Geometry: final body of the model. Coordinates: model frame, mm. A direction names the side the tool comes from. Round coordinates to 2 decimals unless told otherwise and drop trailing zeros. Loops run counter-clockwise (first coordinate to the right, second up) from the corner with the lowest first, then second, coordinate; pieces in that order, holes last. Notation, with made-up numbers: (26, 6) - (63, 6) arc R16 cw to (63, 16) - close; hole circle Ø5 at (-9.5, 58). An arc over 180 degrees is marked (long way). Write item = value, one per line. Start each with the question number.
Item 1: Section A-A (x = 6). Return loops of the section in (y, z), plus the area to 3 significant figures.
Item 2: Draft query along Z for faces 1 (the flat face through (2, -5, 2.2)), 2 (the flat face through (-3, -6, 1.8)), 3 (the cylindrical face through (0.06, 7.15, 0.89)). Return one class per face: pulls with the +Z half, pulls with the -Z half, needs draft (parallel to the pull), parting line crosses it, or undercut.
Item 3: Section D-D (y = 0). Return loops of the section in (x, z).
Item 4: Access query for faces 4 (the flat face through (6.656, -4.209, 0.887)), 5 (the cylindrical face through (2.4, -4.5, 3.8)), 6 (the cylindrical face through (-5, -3.83, 6.04)). Directions: +Z, -Z, +X, -X, +Y, -Y. A direction counts if a zero-diameter tool reaches every point of the face in a straight line with its end or side. Return the directions, or none.
Item 5: Line query: line 1 (Z direction, x = -5.5, y = 2.25); line 2 (Z direction, x = -6.25, y = -4); line 3 (Y direction, x = -8.5, z = 1.25). Output: solid intervals per line, ascending. Write a range as from..to.
Item 6: Section B-B (y = 5.75). Return loops of the section in (x, z) (3 decimals), plus the area to 3 significant figures.
Item 7: Section C-C (x = 0). Return loops of the section in (y, z).
from build123d import *

# Parameters (mm, degrees)
PAD_DEPTH    = 1.8
SKETCH001_R  = 6.3
PAD001_DEPTH = 0.4
SKETCH002_R  = 5.1
PAD002_DEPTH = 3.3
SKETCH003_R  = 6.3
PAD003_DEPTH = 1.1


with BuildPart() as part:
    # Sketch → Pad (new body)
    with BuildSketch(Plane.XY):
        with BuildLine():
            ThreePointArc((3.885224, 6.002294), (0, 7.15), (-3.885224, 6.002294))
            Line((-9.35, 2.465), (-3.885224, 6.002294))
            Line((-9.35, -2.465), (-9.35, 2.465))
            Line((-3.885224, -6.002294), (-9.35, -2.465))
            ThreePointArc((-3.885224, -6.002294), (0, -7.15), (3.885224, -6.002294))
            Line((9.35, -2.465), (3.885224, -6.002294))
            Line((9.35, 2.465), (9.35, -2.465))
            Line((3.885224, 6.002294), (9.35, 2.465))
        make_face()
    extrude(amount=PAD_DEPTH)

    # Sketch001 (on Face5 of Pad003) → Pad001 (join)
    with BuildSketch(Plane.XY.offset(1.8)):
        Circle(SKETCH001_R)
    extrude(amount=PAD001_DEPTH)

    # Sketch002 (on Face12 of Pad001) → Pad002 (join)
    with BuildSketch(Plane.XY.offset(2.2)):
        Circle(SKETCH002_R)
    extrude(amount=PAD002_DEPTH)

    # Sketch003 (on Face14 of Pad002) → Pad003 (join)
    with BuildSketch(Plane.XY.offset(5.5)):
        Circle(SKETCH003_R)
    extrude(amount=PAD003_DEPTH)


solid = part.part
Taken from the geometry:
q1.outline = (-4.63, 0) - (4.63, 0) - (4.63, 1.8) - (1.92, 1.8) - (1.92, 2.2) - (-1.92, 2.2) - (-1.92, 1.8) - (-4.63, 1.8) - close; (-1.92, 5.5) - (1.92, 5.5) - (1.92, 6.6) - (-1.92, 6.6) - close
q1.area = 22.4 mm^2
q2.face_1 = undercut
q2.face_2 = pulls with the +Z half
q2.face_3 = needs draft
q3.outline = (-9.35, 0) - (9.35, 0) - (9.35, 1.8) - (6.3, 1.8) - (6.3, 2.2) - (5.1, 2.2) - (5.1, 5.5) - (6.3, 5.5) - (6.3, 6.6) - (-6.3, 6.6) - (-6.3, 5.5) - (-5.1, 5.5) - (-5.1, 2.2) - (-6.3, 2.2) - (-6.3, 1.8) - (-9.35, 1.8) - close
q4.face_4 = +Z, -Z, +X, -Y
q4.face_5 = none
q4.face_6 = +Z
q5.line_1 = 0..2.2, 5.5..6.6
q5.line_2 = 0..1.8
q5.line_3 = -3.02..3.02
q6.outline = (-4.275, 0) - (4.275, 0) - (4.275, 1.8) - (2.574, 1.8) - (2.574, 2.2) - (-2.574, 2.2) - (-2.574, 1.8) - (-4.275, 1.8) - close; (-2.574, 5.5) - (2.574, 5.5) - (2.574, 6.6) - (-2.574, 6.6) - close
q6.area = 23.1 mm^2
q7.outline = (-7.15, 0) - (7.15, 0) - (7.15, 1.8) - (6.3, 1.8) - (6.3, 2.2) - (5.1, 2.2) - (5.1, 5.5) - (6.3, 5.5) - (6.3, 6.6) - (-6.3, 6.6) - (-6.3, 5.5) - (-5.1, 5.5) - (-5.1, 2.2) - (-6.3, 2.2) - (-6.3, 1.8) - (-7.15, 1.8) - close
